Autodesk Fusion 360 part; units mm, degrees
sketch "Sketch1" plane through (0, 0, 0) normal (0, 0, 1) x (1, 0, 0)
  line L0 (0, 0) -> (-140, 0)
  line L1 (-140, 0) -> (-140, 52)
  line L2 (-140, 52) -> (0, 52)
  line L3 (0, 52) -> (0, 0)
  line L4 (0, -5) -> (-140, -5)
  line L5 (-145, 0) -> (-145, 52)
  line L6 (-140, 57) -> (0, 57)
  line L7 (5, 52) -> (5, 0)
  line L8 (-63, 19) -> (-77, 19)
  line L9 (-58, 28) -> (-58, 24)
  arc A0 (-77, 33) -> (-82, 28) centre (-77, 28) ccw
  arc A1 (-82, 24) -> (-77, 19) centre (-77, 24) ccw
  arc A2 (-63, 19) -> (-58, 24) centre (-63, 24) ccw
  line L10 (-82, 24) -> (-82, 28)
  line L11 (-77, 33) -> (-63, 33)
  arc A3 (-58, 28) -> (-63, 33) centre (-63, 28) ccw
  arc A4 (0, -5) -> (5, 0) centre (0, 0) ccw
  arc A5 (5, 52) -> (0, 57) centre (0, 52) ccw
  arc A6 (-140, 57) -> (-145, 52) centre (-140, 52) ccw
  arc A7 (-145, 0) -> (-140, -5) centre (-140, 0) ccw
  point P0 (-82, 19)
  point P1 (-82, 33)
  point P2 (-58, 33)
  dimension "d1" = 140
  dimension "d2" = 52
  dimension "d4" = 24
  dimension "d5" = 14
  dimension "d7" = 5
  dimension "d8" = 5
  dimension "d9" = 19
  dimension "d10" = 58
  dimension "d11" = 5
extrude "Extrude1" add sketch "Sketch1" along normal blind 10 contours L0 L1 L2 L3
fillet "Fillet1" radius 5 8 edges at (-82, 26, 0) (-80.5355, 31.5355, 0) (-70, 33, 0) (-59.4645, 31.5355, 0) (-58, 26, 0) (-59.4645, 20.4645, 0) (-70, 19, 0) (-80.5355, 20.4645, 0)
extrude "Extrude2" add sketch "Sketch1" along normal blind 2 contours L4 L5 L6 L7 A4 A5 A6 A7
properties part number "Back Plate"
Can you work these out from the model? Positions are in its coordinate system, mm. A direction names the side the tool comes from. Give positions to 0.01 mm unless a question says otherwise; leave off trailing zeros. Order: outer loops, then holes, each group sorted by start corner. A loop starts at its lowest first (then second) coordinate and runs counter-clockwise, first axis right, second up. Notation, with made-up numbers: (61.5, 49) - (101.5, 49) arc R34 cw to (101.5, 80) - close; hole circle Ø1 at (20, 29.5). An arc over 180 degrees is marked (long way). Use a Markdown table: item, result. Add a question column.
Q1. If we section it at A-A on z = 6.75: Write out the boundary of the cut face in (x, y).
Q2. I'm going to push flat-ended pins straight in: pin 1 (5 mm diameter, centred on x = -81.5, y = 45, fed in from -Z); pin 2 (4.5 mm diameter, centred on y = 26, z = 8, fed in from -X); pin 3 (2.5 mm diameter, centred on x = -87, z = 8, fed in from +Y); pin 4 (8 mm diameter, centred on x = -63.5, y = 25.5, fed in from -Z). Where does each tip first touch, or does it pass through?
Q3. If we section it at B-B on y = 10: Write out the boundary of the cut face in (x, z).
Q4. Please list where these lines run through material, in increasing order: line 1 along Y through (x, z) = (-34.5, 4.5); line 2 along X through (y, z) = (10.5, 9.75); line 3 along X through (y, z) = (31, 8).
Q5. If we mould it in two halves opening along X, with no side actions, what happens to faces 4 (the flat face through (-70, 19, 7)), 5 (the flat face through (-71, 38, 10)), 6 (the cylindrical face through (-70, 18, 2)), 7 (the flat face through (-140, 26, 6))? For each: released by +X, released by -X, zero draft, split by the parting line, or undercut.
Q6. On a 3-axis mill with a long thin cutter (end or side, diameter ignored), from which of +Z, -Z, +X, -X, +Y, -Y can I reach the whole of each face in a straight line? I mean faces 1 (the cylindrical face through (-70, 34, 2)), 2 (the flat face through (-71, 52, 6)), 3 (the cylindrical face through (-80, 20, 7)). Say none if no direction works.
Q7. If we section it at C-C on x = -18: Write out the boundary of the cut face in (y, z), plus the area to 3 significant figures.
Answers follow:
| question | item | result |
|---|---|---|
| 1 | outline | (-140, 0) - (0, 0) - (0, 52) - (-140, 52) - close; hole (-82, 24) arc R5 ccw to (-77, 19) - (-63, 19) arc R5 ccw to (-58, 24) - (-58, 28) arc R5 ccw to (-63, 33) - (-77, 33) arc R5 ccw to (-82, 28) - close |
| 2 | pin 1 | stops at z = 0 |
| 2 | pin 2 | stops at x = -140 |
| 2 | pin 3 | stops at y = 52 |
| 2 | pin 4 | passes through |
| 3 | outline | (-145, 0) - (5, 0) - (5, 2) - (0, 2) - (0, 10) - (-140, 10) - (-140, 2) - (-145, 2) - close |
| 4 | line 1 | y = 0 to 52 |
| 4 | line 2 | x = -140 to 0 |
| 4 | line 3 | x = -140 to -81, -59 to 0 |
| 5 | face 4 | undercut |
| 5 | face 5 | zero draft |
| 5 | face 6 | undercut |
| 5 | face 7 | released by -X |
| 6 | face 1 | -Z |
| 6 | face 2 | +Z, +X, -X, +Y |
| 6 | face 3 | +Z, -Z |
| 7 | outline | (-5, 0) - (57, 0) - (57, 2) - (52, 2) - (52, 10) - (0, 10) - (0, 2) - (-5, 2) - close |
| 7 | area | 540 mm^2 |
